Here's how the part is built. I have some questions about the finished solid (model axes, mm). A direction names the side the tool comes from. Coordinates: 2 decimals unless noted, no trailing zeros. Write each loop counter-clockwise with the first axis right and the second up, starting at its lowest first coordinate (ties: lowest second). Pieces come first, ordered by that corner, then holes. Notation, with made-up numbers: (55, 58.25) -> (100, 58.25) arc R14 cw to (100, 66.25) -> close; hole circle Ø4 at (79.5, 79). An arc over 180 degrees is marked (long way). Answer in a Markdown table with one row per item. Add a question column.
from build123d import *

# Parameters (mm, degrees)
F0_W     = 13.1360664964
F0_H     = 63.5863877833
F1_DEPTH = 200
F3_D     = 5
F3_DEPTH = 12
F3_TIP   = 1.5021515476
F5_D     = 5
F5_DEPTH = 12
F5_TIP   = 1.5021515476
F6_W     = 183.091968298
F6_H     = 48.0650532991
F7_DEPTH = 25


with BuildPart() as f1:
    # F0 (on Front) → F1 (new body)
    with BuildSketch(Plane.XZ):
        with Locations((-61.7326833308, -6.2711592764)):
            Rectangle(F0_W, F0_H)
    extrude(amount=F1_DEPTH)

    # F3
    with Locations(Plane.XY.offset(25.5220346153)):
        with Locations((-63.0798041821, -168.1778728962), (-62.9759728909, -98.3595103025), (-62.5574141741, -27.9654413462)):
            Hole(F3_D / 2, depth=F3_DEPTH)
            with Locations((0, 0, -(F3_DEPTH + F3_TIP / 2))):  # 118° drill point
                Cone(0, F3_D / 2, F3_TIP, mode=Mode.SUBTRACT)

    # F5
    with Locations(Plane(origin=(0, 0, 0), x_dir=(1, 0, 0), z_dir=(0, 1, 0))):
        with Locations((-60.7005506754, -12.1290553361), (-61.6644993424, 25.6001017988)):
            Hole(F5_D / 2, depth=F5_DEPTH)
            with Locations((0, 0, -(F5_DEPTH + F5_TIP / 2))):  # 118° drill point
                Cone(0, F5_D / 2, F5_TIP, mode=Mode.SUBTRACT)

    # F6 (on face) → F7 (cut)
    with BuildSketch(Plane.YZ.offset(-55.1646500826)):
        with Locations((-100.3695875406, -6.1469888315)):
            Rectangle(F6_W, F6_H)
    extrude(amount=-F7_DEPTH, mode=Mode.SUBTRACT)


solid = f1.part
Q1. If we mould it in two halves opening along Z, with no side actions, what happens to faces 4 (the flat face through (-62, -99, -38.064)), 5 (the cylindrical face through (-60.71, -26.28, 21.65)), 6 (the cylindrical face through (-63.01, -4.47, 13.09))? For each: pulls with the +Z half, pulls with the -Z half, needs draft (parallel to the pull), parting line crosses it, or undercut.
Q2. Imagine slicing it at C-C on z = 22. Please give me the cut outline in (x, y), plus the area to 3 significant figures.
Q3. Imagine slicing it at B-B on y = -140.5. Please give me the cut outline in (x, z), plus the area to 3 significant figures.
Q4. I'm going to push flat-ended pins straight in: P1, Ø4.5, axis at x = -62.98, y = -98.36, coming from the +Z side; P2, Ø4.5, axis at x = -60.7, z = 12.13, coming from the +Y side. Where does each tip first touch, or does it pass through?
Q5. For faces 1 (the flat face through (-62, -102, -30.18)), 2 (the cylindrical face through (-59.167, -4.474, -25.71)), 3 (the cylindrical face through (-61.237, -166.488, 21.65)), which set-ups out of +Z, -Z, +X, -X, +Y, -Y let a thin tool reach every point of the face, with its end or its side?
Q6. I need wall thicknesses on line 1 (Z direction, x = -58.25, y = -190); line 2 (Y direction, x = -63.5, z = -3); line 3 (X direction, y = -7.5, z = -25.5). Which ranges of each line are inside material? Lowest first, please. Write a range as [from, to].
Q7. Imagine slicing it at A-A on z = -20.5. Please give me the cut outline in (x, y), plus the area to 3 significant figures.
Result sheet:
| question | item | result |
|---|---|---|
| 1 | face 4 | pulls with the -Z half |
| 1 | face 5 | needs draft |
| 1 | face 6 | undercut |
| 2 | outline | (-68.3, -200) -> (-55.16, -200) -> (-55.16, 0) -> (-68.3, 0) -> close; hole circle Ø5 at (-63.08, -168.18); hole circle Ø5 at (-62.98, -98.36); hole circle Ø5 at (-62.56, -27.97) |
| 2 | area | 2,570 mm^2 |
| 3 | outline | (-68.3, -38.06) -> (-55.16, -38.06) -> (-55.16, -30.18) -> (-68.3, -30.18) -> close; (-68.3, 17.89) -> (-55.16, 17.89) -> (-55.16, 25.52) -> (-68.3, 25.52) -> close |
| 3 | area | 204 mm^2 |
| 4 | P1 | stops at z = -30.18 |
| 4 | P2 | stops at y = -191.92 |
| 5 | face 1 | +X, -X |
| 5 | face 2 | +Y |
| 5 | face 3 | +Z |
| 6 | line 1 | z = [-38.06, -30.18], [17.89, 25.52] |
| 6 | line 2 | y = [-200, -191.92], [-8.82, 0] |
| 6 | line 3 | x = [-68.3, -64.16], [-59.17, -55.16] |
| 7 | outline | (-68.3, -200) -> (-55.16, -200) -> (-55.16, -191.92) -> (-68.3, -191.92) -> close; (-68.3, -8.82) -> (-55.16, -8.82) -> (-55.16, 0) -> (-68.3, 0) -> close |
| 7 | area | 222 mm^2 |
